Source: CAD feature listing. Evaluate the final solid. Frame: model axes, mm. A direction names the side the tool comes from. Coordinates: 2 decimals unless noted, no trailing zeros. Write each loop counter-clockwise with the first axis right and the second up, starting at its lowest first coordinate (ties: lowest second). Pieces come first, ordered by that corner, then holes. Notation, with made-up numbers: (77, 74) - (133, 74) arc R23 ccw to (133, 98) - close; hole circle Ø10 at (24, 6). An arc over 180 degrees is marked (long way). One line per item, written item: value.
from build123d import *

# Parameters (mm, degrees)
SKETCH1_W           = 13.2
SKETCH1_H           = 7.9
BOSS_EXTRUDE1_DEPTH = 9.5
SKETCH2_W           = 0.8
SKETCH2_H           = 2
BOSS_EXTRUDE2_DEPTH = 4


with BuildPart() as part:
    # Sketch1 → Boss-Extrude1 (new body)
    with BuildSketch(Plane(origin=(0, 0, 0), x_dir=(1, 0, 0), z_dir=(0, 1, 0))):
        Rectangle(SKETCH1_W, SKETCH1_H)
    extrude(amount=BOSS_EXTRUDE1_DEPTH)

    # Sketch2 → Boss-Extrude2 (add)
    with BuildSketch(Plane.XZ):
        Rectangle(SKETCH2_W, SKETCH2_H)
        with Locations((4.7, 0)):
            Rectangle(SKETCH2_W, SKETCH2_H)
        with Locations((-4.7, 0)):
            Rectangle(SKETCH2_W, SKETCH2_H)
    extrude(amount=BOSS_EXTRUDE2_DEPTH)


solid = part.part
1) Material intervals for line 1 (X direction, y = -1, z = 0.25); line 2 (Y direction, x = -3.25, z = -2.75); line 3 (Z direction, x = -4.5, y = -1.5), sorted ascending.
Values found:
line 1: -5.1 to -4.3, -0.4 to 0.4, 4.3 to 5.1
line 2: 0 to 9.5
line 3: -1 to 1
2) Contact query for flat-ended pins moving along their axis: P1, Ø1.6, axis at y = -1.5, z = 0.5, coming from the -X side; P2, Ø1, axis at y = -2.5, z = 0, coming from the +X side; P3, Ø0.9, axis at x = 0, y = -3, coming from the -Z side. Output: stop coordinate, or through.
Values found:
P1: x = -5.1
P2: x = 5.1
P3: z = -1
3) Section query A-A on z = -0.75. Output: boundary loops of the cut face in (x, y).
Values found:
outline: (-6.6, 0) - (-5.1, 0) - (-5.1, -4) - (-4.3, -4) - (-4.3, 0) - (-0.4, 0) - (-0.4, -4) - (0.4, -4) - (0.4, 0) - (4.3, 0) - (4.3, -4) - (5.1, -4) - (5.1, 0) - (6.6, 0) - (6.6, 9.5) - (-6.6, 9.5) - close
4) Reachability of faces 5 (the flat face through (-4.7, -2, 1)), 6 (the flat face through (4.7, -2, -1)), 7 (the flat face through (-4.3, -2, 0)) from +Z, -Z, +X, -X, +Y, -Y: full face, straight path, thin tool, end or side. Return the list, or none.
Values found:
face 5: +Z, +X, -X, -Y
face 6: -Z, +X, -X, -Y
face 7: +Z, -Z, -Y
5) Draft query along X for faces 1 (the flat face through (-6.6, 5, 0)), 2 (the flat face through (4.3, -2, 0)), 3 (the flat face through (0.4, -2, 0)), 4 (the flat face through (-4.7, -4, 0)). Return one class per face: released by +X, released by -X, zero draft, split by the parting line, or undercut.
Values found:
face 1: released by -X
face 2: undercut
face 3: undercut
face 4: zero draft
6) Section query C-C on z = -2.5. Output: boundary loops of the cut face in (x, y).
Values found:
outline: (-6.6, 0) - (6.6, 0) - (6.6, 9.5) - (-6.6, 9.5) - close
7) Section query B-B on x = 3.25. Output: boundary loops of the cut face in (y, z), then the cut area to 4 significant figures.
Values found:
outline: (0, -3.95) - (9.5, -3.95) - (9.5, 3.95) - (0, 3.95) - close
area: 75.05 mm2
